from build123d import *

# Parameters (mm, degrees)
REVOLU_O2_ANGLE          = 180
ESBO_O4_R                = 10
RESSALTO_EXTRUS_O1_DEPTH = 35
RESSALTO_EXTRUS_O2_DEPTH = 20
ESBO_O8_R                = 3.5
CORTE_EXTRUS_O2_DEPTH    = 20
PADR_OCIRCULAR1_COUNT    = 6
ESBO_O6_R                = 3.5
CORTE_EXTRUS_O1_DEPTH    = 15
ESBO_O9_R                = 1.25
CORTE_EXTRUS_O3_DEPTH    = 6
ESBO_O10_W               = 3
ESBO_O10_H               = 120
CORTE_EXTRUS_O4_DEPTH    = 4.5
ESBO_O11_W               = 3
ESBO_O11_H               = 116.4
RESSALTO_EXTRUS_O5_DEPTH = 2
ESBO_O12_R               = 3.25
RESSALTO_EXTRUS_O6_DEPTH = 20
ESBO_O13_R               = 3
RESSALTO_EXTRUS_O7_DEPTH = 20
CORTE_EXTRUS_O5_DEPTH    = 80.8
ESBO_O16_R               = 93
CORTE_EXTRUS_O6_DEPTH    = 10
ESBO_O17_R               = 93.112429775
ESBO_O17_R_2             = 90.112429775
CORTE_EXTRUS_O7_DEPTH    = 2.5
ESBO_O18_W               = 100
ESBO_O18_H               = 17.238697901
CORTE_EXTRUS_O8_DEPTH    = 15
RESSALTO_EXTRUS_O9_DEPTH = 15


with BuildPart() as part:
    # Esboço3 → Revolução2 (revolve)
    with BuildSketch(Plane.XY):
        with BuildLine():
            Line((97.5, 79.8), (97.5, 11.304491341))
            Line((97.5, 11.304491341), (97.5, 0))
            Line((97.5, 0), (97.5, -40.2))
            Line((97.5, -40.2), (87.5, -40.2))
            Line((87.5, -40.2), (87.5, 0))
            Line((87.5, 0), (60.342408243, 0))
            Line((60.342408243, 0), (60.342408243, 2.95))
            Line((60.342408243, 2.95), (52, 2.95))
            Line((52, 2.95), (44, 10.95))
            Line((44, 10.95), (31, 10.95))
            Line((31, 10.95), (31, 13.7))
            Line((31, 13.7), (22.6, 13.7))
            Line((22.6, 13.7), (22.6, 17))
            Line((22.6, 17), (19.3, 17))
            Line((19.3, 17), (19.3, 17.7))
            Line((19.3, 17.7), (15.3, 17.7))
            Line((15.3, 17.7), (15.3, 21.05))
            Line((15.3, 21.05), (19.3, 21.05))
            Line((19.3, 21.05), (19.3, 21.2))
            Line((19.3, 21.2), (27.626549127, 25.96))
            Line((27.626549127, 25.96), (31.3, 25.96))
            Line((31.3, 25.96), (31.3, 43.96))
            Line((31.3, 43.96), (32.3, 44.96))
            Line((32.3, 44.96), (38.8, 44.96))
            Line((38.8, 44.96), (38.8, 26.9))
            Line((38.8, 26.9), (55.5, 10.2))
            Line((55.5, 10.2), (83.5, 10.2))
            ThreePointArc((83.5, 10.2), (86.328427125, 11.371572875), (87.5, 14.2))
            Line((87.5, 14.2), (87.5, 76.2))
            Line((87.5, 76.2), (93, 76.2))
            Line((93, 76.2), (93, 79.8))
            Line((93, 79.8), (97.5, 79.8))
        make_face()
    revolve(axis=Axis((0, -3.322055656, 0), (0, 1, 0)), revolution_arc=REVOLU_O2_ANGLE)

    # Esboço4 → Ressalto-extrusão1 (add)
    with BuildSketch(Plane(origin=(0, 79.8, 0), x_dir=(1, 0, 0), z_dir=(0, 1, 0))):
        with Locations((70.71, 70.71)):
            Circle(ESBO_O4_R)
        with Locations((-70.71, 70.71)):
            Circle(ESBO_O4_R)
    extrude(amount=-RESSALTO_EXTRUS_O1_DEPTH)

    # Esboço5 → Ressalto-extrusão2 (add)
    with BuildSketch(Plane.XZ.offset(40.2)):
        with BuildLine():
            Line((10, -105), (10, -96.985823706))
            Line((10, -96.985823706), (-10, -96.985823706))
            Line((-10, -96.985823706), (-10, -105))
            ThreePointArc((-10, -105), (0, -115), (10, -105))
        make_face()
    ressalto_extrus_o2 = extrude(amount=-RESSALTO_EXTRUS_O2_DEPTH)

    # Esboço8 → Corte-extrusão2 (cut)
    with BuildSketch(Plane.XZ.offset(40.2)):
        with Locations((0, -105)):
            Circle(ESBO_O8_R)
    corte_extrus_o2 = extrude(amount=-CORTE_EXTRUS_O2_DEPTH, mode=Mode.SUBTRACT)

    # PadrãoCircular1: Ressalto-extrusão2, Corte-extrusão2 ×6 about axis, 3 skipped
    padr_ocircular1_axis = Axis((0, 0, 0), (0, 1, 0))
    add([ressalto_extrus_o2.rotate(padr_ocircular1_axis, i * 360 / PADR_OCIRCULAR1_COUNT) for i in range(1, PADR_OCIRCULAR1_COUNT) if i not in (2, 3, 4)])
    add([corte_extrus_o2.rotate(padr_ocircular1_axis, i * 360 / PADR_OCIRCULAR1_COUNT) for i in range(1, PADR_OCIRCULAR1_COUNT) if i not in (2, 3, 4)], mode=Mode.SUBTRACT)

    # Esboço6 → Corte-extrusão1 (cut)
    with BuildSketch(Plane(origin=(0, 79.8, 0), x_dir=(1, 0, 0), z_dir=(0, 1, 0))):
        with Locations((70.71, 70.71)):
            Circle(ESBO_O6_R)
        with Locations((-70.71, 70.71)):
            Circle(ESBO_O6_R)
    extrude(amount=-CORTE_EXTRUS_O1_DEPTH, mode=Mode.SUBTRACT)

    # Esboço9 → Corte-extrusão3 (cut)
    with BuildSketch(Plane.XZ.offset(-13.7)):
        with Locations((18.738329701, -18.738329701)):
            Circle(ESBO_O9_R)
        with Locations((-18.738329701, -18.738329701)):
            Circle(ESBO_O9_R)
    extrude(amount=-CORTE_EXTRUS_O3_DEPTH, mode=Mode.SUBTRACT)

    # Esboço10 → Corte-extrusão4 (cut)
    with BuildSketch(Plane.XY):
        with Locations((91.5, 19.8)):
            Rectangle(ESBO_O10_W, ESBO_O10_H)
    extrude(amount=-CORTE_EXTRUS_O4_DEPTH, mode=Mode.SUBTRACT)

    # Esboço11 → Ressalto-extrusão5 (add)
    with BuildSketch(Plane.XY):
        with Locations((-91.5, 18)):
            Rectangle(ESBO_O11_W, ESBO_O11_H)
    extrude(amount=RESSALTO_EXTRUS_O5_DEPTH)

    # Esboço12 → Ressalto-extrusão6 (add)
    with BuildSketch(Plane.XY):
        with BuildLine():
            Line((-100.75, 29.8), (-87.5, 29.8))
            Line((-87.5, 29.8), (-87.5, 9.8))
            Line((-87.5, 9.8), (-100.75, 9.8))
            ThreePointArc((-100.75, 9.8), (-110.75, 19.8), (-100.75, 29.8))
        make_face()
        with Locations((-100.75, 19.8)):
            Circle(ESBO_O12_R, mode=Mode.SUBTRACT)
    extrude(amount=-RESSALTO_EXTRUS_O6_DEPTH)

    # Esboço13 → Ressalto-extrusão7 (add)
    with BuildSketch(Plane.XY):
        with BuildLine():
            Line((100.75, 29.8), (93, 29.8))
            Line((93, 29.8), (93, 9.8))
            Line((93, 9.8), (100.75, 9.8))
            ThreePointArc((100.75, 9.8), (110.75, 19.8), (100.75, 29.8))
        make_face()
        with Locations((100.75, 19.8)):
            Circle(ESBO_O13_R, mode=Mode.SUBTRACT)
    extrude(amount=-RESSALTO_EXTRUS_O7_DEPTH)

    # Esboço14 → Corte-extrusão5 (cut, through all)
    with BuildSketch(Plane(origin=(0, 0, 0), x_dir=(-1, 0, 0), z_dir=(0, -1, 0))):
        with BuildLine():
            ThreePointArc((34.350508428, 67.496062714), (0, 70), (-34.350508428, 67.496062714))
            ThreePointArc((-34.350508428, 67.496062714), (-47.016691783, 50.479370931), (-30, 37.813187576))
            ThreePointArc((-30, 37.813187576), (0, 40), (30, 37.813187576))
            ThreePointArc((30, 37.813187576), (47.016691783, 50.479370931), (34.350508428, 67.496062714))
        make_face()
    extrude(amount=-CORTE_EXTRUS_O5_DEPTH, mode=Mode.SUBTRACT)

    # Esboço16 → Corte-extrusão6 (cut)
    with BuildSketch(Plane(origin=(0, 76.2, 0), x_dir=(1, 0, 0), z_dir=(0, 1, 0))):
        Circle(ESBO_O16_R)
    extrude(amount=CORTE_EXTRUS_O6_DEPTH, mode=Mode.SUBTRACT)

    # Esboço17 → Corte-extrusão7 (cut)
    with BuildSketch(Plane.XZ.offset(40.2)):
        Circle(ESBO_O17_R)
        Circle(ESBO_O17_R_2, mode=Mode.SUBTRACT)
    extrude(amount=-CORTE_EXTRUS_O7_DEPTH, mode=Mode.SUBTRACT)

    # Esboço18 → Corte-extrusão8 (cut, symmetric)
    with BuildSketch(Plane(origin=(0, -20.1, 0), x_dir=(-1, 0, 0), z_dir=(0, -1, 0))):
        with Locations((0, 72.662310295)):
            Rectangle(ESBO_O18_W, ESBO_O18_H)
    extrude(amount=CORTE_EXTRUS_O8_DEPTH, both=True, mode=Mode.SUBTRACT)

    # Esboço19 → Ressalto-extrusão9 (add, symmetric)
    with BuildSketch(Plane(origin=(0, -20.1, 0), x_dir=(-1, 0, 0), z_dir=(0, -1, 0))):
        with BuildLine():
            Line((32.396633626, 81.281659245), (-32.396633626, 81.281659245))
            ThreePointArc((-32.396633626, 81.281659245), (0, 87.5), (32.396633626, 81.281659245))
        make_face()
    extrude(amount=RESSALTO_EXTRUS_O9_DEPTH, both=True)


solid = part.part
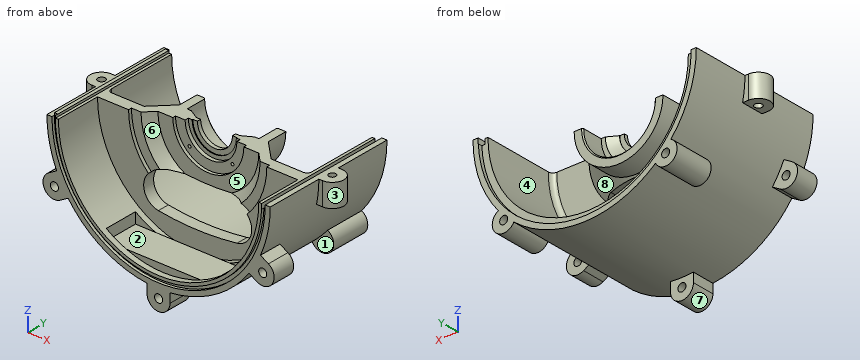
Source: CAD feature listing. Evaluate the final solid. Frame: model axes, mm. Face numbers are marked on the shaded views. A direction names the side the tool comes from. Give positions to 0.01 mm unless a question says otherwise; leave off trailing zeros. Write each loop counter-clockwise with the first axis right and the second up, starting at its lowest first coordinate (ties: lowest second). Pieces come first, ordered by that corner, then holes. Notation, with made-up numbers: M -17.75,32 L -4.75,32 A7 ccw -4.75,42 Z; hole C -28,-34.5 d6. An arc over 180 degrees is marked long. Answer as a JSON object with one key per item and string values.
Q1. Ray query, line 1 along X through (y, z) = (54, -76.5); line 2 along X through (y, z) = (24.5, -15); line 3 along Z through (x, y) = (30.5, 25.5). Return the intervals inside material, ascending.
Geometry check:
{"line 1": "x = -78.86 to -62.56, -60.45 to -42.47, 42.47 to 60.45, 62.56 to 78.86", "line 2": "x = -109.58 to -86.2, -38.37 to -20.09, 20.09 to 38.37, 86.2 to 109.58", "line 3": "z = -92.61 to -82.01, -26.19 to 0"}
Q2. Cut plane D-D, the plane y = 55. Return the cut outline in (x, z), then the cut area to 3 significant figures.
Geometry check:
{"outline": "M -97.5,0 A97.5 ccw -75.36,-61.86 A10 ccw long -61.86,-75.36 A97.5 ccw 61.86,-75.36 A10 ccw long 75.36,-61.86 A97.5 ccw 97.5,0 L 93,0 L 93,-4.5 L 90,-4.5 L 90,0 L 87.5,0 A87.5 cw -87.5,0 L -90,0 L -90,2 L -93,2 L -93,0 Z", "area": "3,320 mm^2"}
Q3. Cut plane B-B, the plane y = -26. Count the separate pieces of the cut face and the enclosed holes in it, then the cut area to 3 significant figures.
Geometry check:
{"separate pieces": "1", "enclosed holes": "3", "area": "3,830 mm^2"}
Q4. Access query for the marked faces 1, 2, 3 and 4. Directions: +Z, -Z, +X, -X, +Y, -Y. A direction counts if a zero-diameter tool reaches every point of the face in a straight line with its end or side. Return the directions, or none.
Geometry check:
{"face 1": "-Z, +X, -Y", "face 2": "+Z", "face 3": "+Z, -Z, +X", "face 4": "+Y"}
Q5. Contact query for flat-ended pins moving along their axis: P1, Ø2, axis at y = 16, z = -86, coming from the +X side; P2, Ø3, axis at y = -26.5, z = -78, coming from the +X side; P3, Ø25, axis at x = -5, z = -9, coming from the +Y side; P4, Ø12, axis at x = 38, z = -47, coming from the +Y side. Output: stop coordinate, or through.
Geometry check:
{"P1": "stops at x = 47.76", "P2": "stops at x = 60.45", "P3": "stops at y = 23.2", "P4": "passes through"}
Q6. Mould query, pull axis Z, two halves, no side actions, for the marked faces 5, 6, 7 and 8. Classes: +Z half, -Z half, draft (parallel to the pull), parting line (faces both ways), or undercut.
Geometry check:
{"face 5": "draft", "face 6": "+Z half", "face 7": "-Z half", "face 8": "undercut"}
Q7. Cut plane A-A, the plane y = 72. Return the cut outline in (x, z), then the cut area to 3 significant figures.
Geometry check:
{"outline": "M -97.5,0 A97.5 ccw -75.36,-61.86 A10 ccw long -61.86,-75.36 A97.5 ccw 61.86,-75.36 A10 ccw long 75.36,-61.86 A97.5 ccw 97.5,0 L 93,0 L 93,-4.5 L 90,-4.5 L 90,0 L 87.5,0 A87.5 cw -87.5,0 L -90,0 L -90,2 L -93,2 L -93,0 Z; hole C -70.71,-70.71 d7; hole C 70.71,-70.71 d7", "area": "3,240 mm^2"}
